Input: part model. Units: mm. Frame: model coordinates. A direction names the side the tool comes from. Coordinates: 2 decimals unless noted, no trailing zeros. Loops run counter-clockwise (first coordinate to the right, second up) from the corner with the lowest first, then second, coordinate; pieces in that order, holes last. Notation, with made-up numbers: M -27,38.25 L -13,38.25 A24 ccw -13,57.25 Z; hole C -37,9.25 d10. An arc over 180 degrees is marked long. Use a Markdown table: item, result. Add a question column.
1. Section B-B on z = -5. Output: boundary loops of the cut face in (x, y).
2. Section D-D on y = -20.75. Output: boundary loops of the cut face in (x, z), then the cut area to 3 significant figures.
3. Draft query along Y for faces 1 (the flat face through (3, -23, -55)), 2 (the cylindrical face through (0.74, -8.368, -48.597)), 3 (the flat face through (44.4, 0, -25)). Return one class per face: +Y half, -Y half, draft (parallel to the pull), parting line (faces both ways), or undercut.
4. Line query: L1, parallel to X at y = 2.6, z = -25; L2, parallel to X at y = 3.2, z = -5; L3, parallel to Z at x = 26.5, y = -4.75. Output: solid intervals per line, ascending. Write a range as [from, to].
5. Pin query (flat end, axial travel): pin 1 (16 mm diameter, centred on x = 31, z = -27, fed in from -Y); pin 2 (2.5 mm diameter, centred on x = 12, y = 3.5, fed in from -Z); pin 3 (10 mm diameter, centred on y = -13.5, z = -49.5, fed in from +X). Return the tip coordinate at first contact, or that it passes through.
6. Set-up query: faces 4 (the flat face through (1, -11, -63)), 5 (the flat face through (27, -1, -31.5)), 6 (the flat face through (9.4, -3, -24)). Return all of +Z, -Z, +X, -X, +Y, -Y with unobstructed straight access to the full face (end or side cutting, diameter ignored); none if empty.
7. Section A-A on z = -27.5. Output: boundary loops of the cut face in (x, y), then the cut area to 3 significant figures.
8. Section C-C on y = -14.75. Output: boundary loops of the cut face in (x, z), then the cut area to 3 significant figures.
```python
from build123d import *

# Parameters (mm, degrees)
SKETCH1_R                = 1.75
SKETCH1_W                = 7.2
SKETCH1_H                = 5.4
BOSS_EXTRUDE1_DEPTH      = 5
FILLET5_RADIUS           = 10
FILLET5_LENGTH           = 5
FILLET2_R                = 5.4
FILLET6_R                = 5.4
SKETCH3_W                = 6
SKETCH3_H                = 13
BOSS_EXTRUDE4_DEPTH      = 5.5
SKETCH5_W                = 23
SKETCH5_H                = 13
CUT_EXTRUDE1_DEPTH       = 3.5
CUT_EXTRUDE2_DEPTH       = 76.201396264
FILLET9_R                = 4
BOSS_EXTRUDE7_DEPTH      = 32
BOSS_EXTRUDE7_DEPTH_BACK = 12
SKETCH7_W                = 10
SKETCH7_H                = 28
FILLET10_R               = 10
SKETCH9_R                = 1
CUT_EXTRUDE4_DEPTH       = 7
SKETCH15_W               = 5
SKETCH15_H               = 32
CUT_EXTRUDE7_DEPTH       = 30
CUT_EXTRUDE8_DEPTH       = 5
CUT_EXTRUDE9_DEPTH       = 3.5
SKETCH22_R               = 1.3
CUT_EXTRUDE10_DEPTH      = 1.5
SKETCH22_3_R             = 2.35
SKETCH22_3_R_2           = 1.3
CUT_EXTRUDE11_DEPTH      = 1
SKETCH23_R               = 0.75
CUT_EXTRUDE12_DEPTH      = 1.75


with BuildPart() as part:
    # Sketch1 → Boss-Extrude1 (new body)
    # profile 1 of 4: a face of its own
    with BuildSketch(Plane(origin=(0, 0, 0), x_dir=(1, 0, 0), z_dir=(0, 1, 0))):
        with BuildLine():
            Line((3.25, 25), (0, 25))
            Line((0, 25), (0, 15))
            Line((0, 15), (10, 0))
            Line((10, 0), (26, 0))
            Line((26, 0), (36, 15))
            Line((36, 15), (60, 15))
            Line((60, 15), (60, 25))
            Line((60, 25), (44.5, 25))
            Line((44.5, 25), (44.5, 19.6))
            Line((44.5, 19.6), (37.3, 19.6))
            Line((37.3, 19.6), (26.5, 19.6))
            Line((26.5, 19.6), (26.5, 25))
            Line((26.5, 25), (6.75, 25))
            ThreePointArc((6.75, 25), (5, 23.25), (3.25, 25))
        make_face()
        with Locations(Location((13, 5, 0), (0, 0, 270))):
            Circle(SKETCH1_R, mode=Mode.SUBTRACT)
        with Locations(Location((23, 5, 0), (0, 0, 270))):
            Circle(SKETCH1_R, mode=Mode.SUBTRACT)
    # profile 2 of 4: a face of its own
    with BuildSketch(Plane(origin=(0, 0, 0), x_dir=(1, 0, 0), z_dir=(0, 1, 0))):
        with BuildLine():
            Line((10, 45), (0, 33.819660113))
            Line((0, 33.819660113), (0, 25))
            Line((0, 25), (3.25, 25))
            ThreePointArc((3.25, 25), (5, 26.75), (6.75, 25))
            Line((6.75, 25), (26.5, 25))
            Line((26.5, 25), (26.5, 30.4))
            Line((26.5, 30.4), (37.3, 30.4))
            Line((37.3, 30.4), (44.5, 30.4))
            Line((44.5, 30.4), (44.5, 25))
            Line((44.5, 25), (60, 25))
            Line((60, 25), (60, 35))
            Line((60, 35), (36, 35))
            Line((36, 35), (26, 45))
            Line((26, 45), (10, 45))
        make_face()
    # profile 3 of 4: a face of its own
    with BuildSketch(Plane(origin=(0, 0, 0), x_dir=(1, 0, 0), z_dir=(0, 1, 0))):
        with Locations((40.9, 27.7)):
            Rectangle(SKETCH1_W, SKETCH1_H)
    # profile 4 of 4: a face of its own
    with BuildSketch(Plane(origin=(0, 0, 0), x_dir=(1, 0, 0), z_dir=(0, 1, 0))):
        with Locations((40.9, 22.3)):
            Rectangle(SKETCH1_W, SKETCH1_H)
    extrude(amount=BOSS_EXTRUDE1_DEPTH)

    # Fillet5: full round fillet: the end face becomes a half cylinder, R = half its width
    fillet5_face = Plane((60, 2.5, -25), x_dir=(0, -1, 0), z_dir=(1, 0, 0))  # on the end face: x along it, z out of the body
    fillet5_slab = fillet5_face.offset(-FILLET5_RADIUS / 2) * Box(FILLET5_LENGTH, 2 * FILLET5_RADIUS, FILLET5_RADIUS, mode=Mode.PRIVATE)  # the body's end, R deep
    fillet5_round = Plane((50, 2.5, -25), x_dir=(1, 0, 0), z_dir=(0, -1, 0)) * Cylinder(FILLET5_RADIUS, FILLET5_LENGTH, mode=Mode.PRIVATE)  # its axis R under the face
    add(fillet5_slab - fillet5_round, mode=Mode.SUBTRACT)

    # Fillet2
    fillet2_edges = [part.edges().sort_by_distance(p)[0] for p in [
        (26.5, 2.5, -30.4),
        (26.5, 2.5, -19.6),
    ]]
    fillet(fillet2_edges, radius=FILLET2_R - 0.0001)  # a hair under: the kernel refuses the full size

    # Fillet6
    fillet6_edges = [part.edges().sort_by_distance(p)[0] for p in [
        (37.3, 2.5, -19.6),
        (37.3, 2.5, -30.4),
    ]]
    fillet(fillet6_edges, radius=FILLET6_R - 0.0001)  # a hair under: the kernel refuses the full size

    # Sketch3 → Boss-Extrude4 (add)
    with BuildSketch(Plane.XZ):
        with Locations((12.4, -25)):
            Rectangle(SKETCH3_W, SKETCH3_H)
        Polygon((38.4, -25), (38.4, -31.5), (44.4, -31.5), (44.4, -18.5), (38.4, -18.5), align=None)
        Polygon((31.9, -31.5), (15.4, -31.5), (9.4, -31.5), (9.4, -35), (36, -35), (44.4, -35), (44.4, -31.5), (38.4, -31.5), align=None)
        Polygon((9.4, -18.5), (15.4, -18.5), (31.9, -18.5), (38.4, -18.5), (44.4, -18.5), (44.4, -15), (36, -15), (9.4, -15), align=None)
    extrude(amount=BOSS_EXTRUDE4_DEPTH)

    # Sketch5 → Cut-Extrude1 (cut)
    with BuildSketch(Plane.XZ):
        with Locations((26.9, -25)):
            Rectangle(SKETCH5_W, SKETCH5_H)
    extrude(amount=-CUT_EXTRUDE1_DEPTH, mode=Mode.SUBTRACT)

    # Sketch6 → Cut-Extrude2 (cut, through all)
    with BuildSketch(Plane.XZ):
        with BuildLine():
            Line((44.4, -15), (44.4, -35))
            Line((44.4, -35), (50, -35))
            ThreePointArc((50, -35), (60, -25), (50, -15))
            Line((50, -15), (44.4, -15))
        make_face()
    extrude(amount=-CUT_EXTRUDE2_DEPTH, mode=Mode.SUBTRACT)

    # Fillet9
    fillet9_edges = [part.edges().sort_by_distance(p)[0] for p in [
        (44.4, -0.25, -35),
        (44.4, -0.25, -15),
    ]]
    fillet(fillet9_edges, radius=FILLET9_R)

    # Sketch7 → Boss-Extrude7 (add, two sides: drawn at the far end of the back side and taken through both)
    with BuildSketch(Plane(origin=(0, 0, -45), x_dir=(-1, 0, 0), z_dir=(0, 0, -1)).offset(-BOSS_EXTRUDE7_DEPTH_BACK)):
        with Locations((-5, -9)):
            Rectangle(SKETCH7_W, SKETCH7_H)
    extrude(amount=BOSS_EXTRUDE7_DEPTH + BOSS_EXTRUDE7_DEPTH_BACK)

    # Fillet10
    fillet10_edges = [part.edges().sort_by_distance(p)[0] for p in [
        (5, 5, -77),
        (5, -23, -33),
        (5, -23, -77),
    ]]
    fillet(fillet10_edges, radius=FILLET10_R)

    # Sketch9 → Cut-Extrude4 (cut)
    with BuildSketch(Plane.XZ.offset(5.5)):
        with Locations(Location((13.1, -25, 0), (0, 0, 270))):
            Circle(SKETCH9_R)
        with Locations(Location((40.7, -25, 0), (0, 0, 270))):
            Circle(SKETCH9_R)
    extrude(amount=-CUT_EXTRUDE4_DEPTH, mode=Mode.SUBTRACT)

    # Sketch15 → Cut-Extrude7 (cut)
    with BuildSketch(Plane(origin=(0, 5, 0), x_dir=(1, 0, 0), z_dir=(0, 1, 0))):
        with Locations((7.5, 61)):
            Rectangle(SKETCH15_W, SKETCH15_H)
    extrude(amount=-CUT_EXTRUDE7_DEPTH, mode=Mode.SUBTRACT)

    # Sketch17 → Cut-Extrude8 (cut)
    with BuildSketch(Plane(origin=(10, 0, 0), x_dir=(0, 0, -1), z_dir=(1, 0, 0))):
        with BuildLine():
            Line((45, -23), (45, 0))
            Line((45, 0), (35, 0))
            Line((35, 0), (35, -5.5))
            Line((35, -5.5), (33, -5.5))
            Line((33, -5.5), (33, -13))
            ThreePointArc((33, -13), (35.928932188, -20.071067812), (43, -23))
            Line((43, -23), (45, -23))
        make_face()
    extrude(amount=-CUT_EXTRUDE8_DEPTH, mode=Mode.SUBTRACT)

    # Sketch8 → Cut-Extrude9 (cut)
    with BuildSketch(Plane(origin=(5, 0, 0), x_dir=(0, 0, -1), z_dir=(1, 0, 0))):
        with BuildLine():
            Line((62.651785714, -5.768708182), (48.8125, -7.260073637))
            ThreePointArc((48.8125, -7.260073637), (47.25, -9), (48.8125, -10.739926363))
            Line((48.8125, -10.739926363), (62.651785714, -12.231291818))
            ThreePointArc((62.651785714, -12.231291818), (66.25, -9), (62.651785714, -5.768708182))
        make_face()
    extrude(amount=-CUT_EXTRUDE9_DEPTH, mode=Mode.SUBTRACT)

    # Sketch22 → Cut-Extrude10 (cut)
    with BuildSketch(Plane.ZY):
        with Locations((-63, -9)):
            Circle(SKETCH22_R)
    extrude(amount=-CUT_EXTRUDE10_DEPTH, mode=Mode.SUBTRACT)

    # Sketch22<3> → Cut-Extrude11 (cut)
    with BuildSketch(Plane.ZY):
        with Locations((-63, -9)):
            Circle(SKETCH22_3_R)
        with Locations((-63, -9)):
            Circle(SKETCH22_3_R_2, mode=Mode.SUBTRACT)
    extrude(amount=-CUT_EXTRUDE11_DEPTH, mode=Mode.SUBTRACT)

    # Sketch23 → Cut-Extrude12 (cut)
    with BuildSketch(Plane.ZY):
        with Locations((-49, -9)):
            Circle(SKETCH23_R)
    extrude(amount=-CUT_EXTRUDE12_DEPTH, mode=Mode.SUBTRACT)


solid = part.part
```
Answers below:
| question | item | result |
|---|---|---|
| 1 | outline | M 6.67,0 L 11.25,0 L 11.25,5 L 6.67,5 Z; M 14.75,0 L 21.25,0 L 21.25,5 L 14.75,5 Z; M 24.75,0 L 29.33,0 L 29.33,5 L 24.75,5 Z |
| 2 | outline | M 0,-73.32 L 5,-73.32 L 5,-36.68 L 0,-36.68 Z |
| 2 | area | 183 mm² |
| 3 | face 1 | -Y half |
| 3 | face 2 | undercut |
| 3 | face 3 | draft |
| 4 | L1 | x = [0, 3.25], [6.75, 15.4], [38.4, 44.4] |
| 4 | L2 | x = [6.67, 11.25], [14.75, 21.25], [24.75, 29.33] |
| 4 | L3 | z = [-35, -31.5], [-18.5, -15] |
| 5 | pin 1 | stops at y = -5.5 |
| 5 | pin 2 | stops at z = -45 |
| 5 | pin 3 | stops at x = 5 |
| 6 | face 4 | -X |
| 6 | face 5 | -Y |
| 6 | face 6 | +Z, -X, -Y |
| 7 | outline | M 0,0 L 9.4,0 L 9.4,-5.5 L 15.4,-5.5 L 15.4,3.5 L 27.11,3.5 L 27.11,5 L 0,5 Z; M 36.69,3.5 L 38.4,3.5 L 38.4,-5.5 L 44.4,-5.5 L 44.4,5 L 36.69,5 Z |
| 7 | area | 193 mm² |
| 8 | outline | M 0,-76.85 L 5,-76.85 L 5,-33.15 L 0,-33.15 Z |
| 8 | area | 218 mm² |
